Geometry: final body of the model. Coordinates: model frame, mm. A direction names the side the tool comes from. Round coordinates to 2 decimals unless told otherwise and drop trailing zeros. Loops run counter-clockwise (first coordinate to the right, second up) from the corner with the lowest first, then second, coordinate; pieces in that order, holes last. Notation, with made-up numbers: (88.5, 17) -> (143.5, 17) arc R30 ccw to (143.5, 50) -> close; hole circle Ø3 at (0, -4.75). An arc over 180 degrees is marked (long way). Answer in a Markdown table with one row per item.
```python
from build123d import *

# Parameters (mm, degrees)
F0_W                 = 8
F0_H                 = 6
F2_SIZE              = 0.3
F5_D                 = 2.5
F5_DEPTH             = 5
F5_CSINK_D           = 5.3
F5_CSINK_ANGLE       = 60
F5_TIP               = 0.7510757738
F5_ON_F4_D           = 2.5
F5_ON_F4_DEPTH       = 5
F5_ON_F4_CSINK_D     = 5.3
F5_ON_F4_CSINK_ANGLE = 60
F5_ON_F4_TIP         = 0.7510757738


with BuildPart() as f1:
    # F0 (on Top) → F1 (revolve)
    with BuildSketch(Plane.XY):
        with Locations((147.5, 3)):
            Rectangle(F0_W, F0_H)
        Polygon((139.5, 7.95), (139.5, 0), (143.5, 0), (143.5, 6), (143.5, 7.95), align=None)
        Polygon((118, 8), (118, 0), (139.5, 0), (139.5, 7.95), (139.5, 8), align=None)
        Polygon((0, 8), (0, 0), (118, 0), (118, 8), (118, 9), (0, 9), align=None)
        Polygon((-21.5, 0), (0, 0), (0, 8), (-21.5, 8), (-21.5, 7.95), align=None)
        Polygon((-25.5, 0), (-21.5, 0), (-21.5, 7.95), (-25.5, 7.95), (-25.5, 6), align=None)
        with Locations((-29.5, 3)):
            Rectangle(F0_W, F0_H)
    revolve(axis=Axis((59, 0, 0), (1, 0, 0)))

    # F2
    f2_edges = [f1.edges().sort_by_distance(p)[0] for p in [
        (151.5, -6, 0),
        (143.5, -7.95, 0),
        (118, -9, 0),
        (0, -9, 0),
        (-25.5, -7.95, 0),
        (-33.5, -6, 0),
    ]]
    chamfer(f2_edges, length=F2_SIZE)

    # F5
    with Locations(Plane(origin=(-33.5, 0, 0), x_dir=(0, -1, 0), z_dir=(-1, 0, 0))):
        with Locations((0, 0)):
            CounterSinkHole(F5_D / 2, F5_CSINK_D / 2, depth=F5_DEPTH, counter_sink_angle=F5_CSINK_ANGLE)
            with Locations((0, 0, -(F5_DEPTH + F5_TIP / 2))):  # 118° drill point
                Cone(0, F5_D / 2, F5_TIP, mode=Mode.SUBTRACT)

    # F5 on F4
    with Locations(Plane.YZ.offset(151.5)):
        with Locations((0, 0)):
            CounterSinkHole(F5_ON_F4_D / 2, F5_ON_F4_CSINK_D / 2, depth=F5_ON_F4_DEPTH, counter_sink_angle=F5_ON_F4_CSINK_ANGLE)
            with Locations((0, 0, -(F5_ON_F4_DEPTH + F5_ON_F4_TIP / 2))):  # 118° drill point
                Cone(0, F5_ON_F4_D / 2, F5_ON_F4_TIP, mode=Mode.SUBTRACT)


solid = f1.part
```
Item 1: First-contact query: P1, Ø2, axis at y = 0, z = 0, coming from the +X side; P2, Ø1.5, axis at x = 127.5, z = -7, coming from the +Y side; P3, Ø4, axis at x = 114.5, z = -3, coming from the +Y side; P4, Ø8.5, axis at y = 0.5, z = -2.5, coming from the +X side. Flat tips, straight axial feed; report the tip coordinate or a pass-through.
Ans:
| item | result |
|---|---|
| P1 | x = 146.35 |
| P2 | y = 4.99 |
| P3 | y = 8.94 |
| P4 | x = 151.5 |
Item 2: Mould query, pull axis Z, two halves, no side actions, for faces 1 (the flat face through (118, -8, -3)), 2 (the cylindrical face through (128.6, -1.73, -7.81)), 3 (the conical face through (-31.46, -0.19, 1.46)). Classes: released by +Z, released by -Z, zero draft, split by the parting line, or undercut.
Ans:
| item | result |
|---|---|
| face 1 | zero draft |
| face 2 | split by the parting line |
| face 3 | undercut |
Item 3: Section query A-A, the plane x = 110. Output: boundary loops of the cut face in (y, z).
Ans:
| item | result |
|---|---|
| outline | circle Ø18 at (0, 0) |
Item 4: Set-up query: faces 4 (the cylindrical face through (141.32, -1.72, -7.76)), 5 (the flat face through (151.5, -2.5, 1.3)), 6 (the cylindrical face through (-10.9, -1.73, -7.81)). Return all of +Z, -Z, +X, -X, +Y, -Y with unobstructed straight access to the full face (end or side cutting, diameter ignored); none if empty.
Ans:
| item | result |
|---|---|
| face 4 | +X |
| face 5 | +Z, -Z, +X, +Y, -Y |
| face 6 | -X |
Item 5: Ray query, L1, parallel to Z at x = 147.8, y = 0; L2, parallel to X at y = 3.75, z = -5; L3, parallel to X at y = 7, z = 4.25. Return the intervals inside material, ascending.
Ans:
| item | result |
|---|---|
| L1 | -6 to -1.25, 1.25 to 6 |
| L2 | -25.5 to 143.5 |
| L3 | 0 to 118 |
